```python
from build123d import *

# Parameters (mm, degrees)
BOSS_EXTRUDE1_DEPTH = 10
FILLET1_R           = 2
FILLET2_RADIUS      = 10
FILLET2_LENGTH      = 1.25
FILLET3_R           = 6
SKETCH2_R           = 4.25
CUT_EXTRUDE1_DEPTH  = 29.94740921


with BuildPart() as part:
    # Sketch1 → Boss-Extrude1 (new, symmetric)
    with BuildSketch(Plane.XY):
        Polygon((0, 1.25), (-1.25, 0), (-27.05, 0), (-27.05, -1.25), (0, -1.25), (1.25, 0), (27.05, 0), (27.05, 1.25), align=None)
    extrude(amount=BOSS_EXTRUDE1_DEPTH, both=True)

    # Fillet1
    fillet1_edges = [part.edges().sort_by_distance(p)[0] for p in [
        (-27.05, -0.625, -10),
        (-27.05, -0.625, 10),
    ]]
    fillet(fillet1_edges, radius=FILLET1_R)

    # Fillet2: full round fillet: the end face becomes a half cylinder, R = half its width
    fillet2_face = Plane((27.05, 0.625, 0), x_dir=(0, -1, 0), z_dir=(1, 0, 0))  # on the end face: x along it, z out of the body
    fillet2_slab = fillet2_face.offset(-FILLET2_RADIUS / 2) * Box(FILLET2_LENGTH, 2 * FILLET2_RADIUS, FILLET2_RADIUS, mode=Mode.PRIVATE)  # the body's end, R deep
    fillet2_round = Plane((17.05, 0.625, 0), x_dir=(1, 0, 0), z_dir=(0, -1, 0)) * Cylinder(FILLET2_RADIUS, FILLET2_LENGTH, mode=Mode.PRIVATE)  # its axis R under the face
    add(fillet2_slab - fillet2_round, mode=Mode.SUBTRACT)

    # Fillet3
    # the kernel refuses this fillet: 6 mm, written as the material it takes off along each edge
    with BuildSketch(Plane(origin=(0, -1.25, -16.039298937), x_dir=(-1, 0, 0), z_dir=(0, 0, 1))) as fillet3_piece_1:
        with BuildLine():
            CenterArc((2.415719575, -6), FILLET3_R, 90, 37.658462006)
            Line((-1.25, -1.25), (-1.323314391, -1.155))
            ThreePointArc((-1.323314391, -1.155), (-0.709852814, -0.540147186), (-0.084852814, 0.084852814))
            Line((-0.084852814, 0.084852814), (0, 0.12))
            Line((0, 0.12), (2.415719575, 0.12))
            Line((2.415719575, 0.12), (2.415719575, 0))
        make_face()
    extrude(amount=32.078597873, mode=Mode.SUBTRACT)
    with BuildSketch(Plane(origin=(0, 1.25, 16.039298937), x_dir=(1, 0, 0), z_dir=(0, 0, -1))) as fillet3_piece_2:
        with BuildLine():
            CenterArc((2.415719575, 6), FILLET3_R, 232.341537994, 37.658462006)
            Line((-1.25, 1.25), (-1.323314391, 1.155))
            ThreePointArc((-1.323314391, 1.155), (-0.709852814, 0.540147186), (-0.084852814, -0.084852814))
            Line((-0.084852814, -0.084852814), (0, -0.12))
            Line((0, -0.12), (2.415719575, -0.12))
            Line((2.415719575, -0.12), (2.415719575, 0))
        make_face()
    extrude(amount=32.078597873, mode=Mode.SUBTRACT)

    # Sketch2 → Cut-Extrude1 (cut, through all)
    with BuildSketch(Plane(origin=(0, 1.25, 0), x_dir=(1, 0, 0), z_dir=(0, 1, 0))):
        with Locations(Location((17.05, 0, 0), (0, 0, 270))):
            Circle(SKETCH2_R)
    extrude(amount=-CUT_EXTRUDE1_DEPTH, mode=Mode.SUBTRACT)


solid = part.part
```
Can you work these out from the model? Positions are in its coordinate system, mm. A direction names the side the tool comes from. Give positions to 0.01 mm unless a question says otherwise; leave off trailing zeros. Loops run counter-clockwise (first coordinate to the right, second up) from the corner with the lowest first, then second, coordinate; pieces in that order, holes last. Notation, with made-up numbers: M 56,39 L 66,39 A13 ccw 66,57 Z; hole C 83.25,-2.75 d10. An arc over 180 degrees is marked long. One line per item, written item: value.
(1) Suppose I cut it at B-B on x = 11. List the corners of the cut face in (y, z) for me.
Returned:
outline: M 0,-10 L 1.25,-10 L 1.25,10 L 0,10 Z
(2) We'd pull the mould along Z, two halves only. Please class faces 4 (the face through (-4.3, -0.3, -10)), 5 (the face through (-26.48, -0.63, 9.4)), 6 (the face through (12, 1.25, 0)), 7 (the face through (21.264, 0.634, -0.553)): released by +Z, released by -Z, zero draft, split by the parting line, or undercut.
Returned:
face 4: released by -Z
face 5: released by +Z
face 6: zero draft
face 7: undercut
(3) Will these pins go through, and if not, where does the flat tip stop? pin 1 (1.5 mm diameter, centred on x = -7, z = 5.5, fed in from +Y); pin 2 (12 mm diameter, centred on x = 2, z = 6.5, fed in from -Y).
Returned:
pin 1: y = 0
pin 2: y = -1.25
(4) Suppose I cut it at C-C on z = -5. List the corners of the cut face in (x, y) for me.
Returned:
outline: M -27.05,-1.25 L -2.42,-1.25 A6 ccw 1.25,0 L 25.71,0 L 25.71,1.25 L 2.42,1.25 A6 ccw -1.25,0 L -27.05,0 Z
(5) I need wall thicknesses on line 1 (Y direction, x = -11.5, z = -6.25); line 2 (Y direction, x = 8.5, z = -9); line 3 (X direction, y = 0.65, z = 0). Which ranges of each line are inside material? Lowest first, please.
Returned:
line 1: -1.25 to 0
line 2: 0 to 1.25
line 3: -0.2 to 12.8, 21.3 to 27.05
(6) Suppose I cut it at A-A on z = 0. List the corners of the cut face in (x, y) for me, plus the area to 3 significant figures.
Returned:
outline: M -27.05,-1.25 L -2.42,-1.25 A6 ccw 1.25,0 L 12.8,0 L 12.8,1.25 L 2.42,1.25 A6 ccw -1.25,0 L -27.05,0 Z; M 21.3,0 L 27.05,0 L 27.05,1.25 L 21.3,1.25 Z
area: 57.2 mm^2
(7) Which directions (+Z, -Z, +X, -X, +Y, -Y) give clear straight access to the entire face, cutting with the end or side of a thin tool? Please do faces 1 (the face through (27.048, 0.616, -0.22)), 2 (the face through (-14, 0, 0)), 3 (the face through (11, 0, 0)).
Returned:
face 1: +X, +Y, -Y
face 2: +Z, -Z, -X, +Y
face 3: +Z, -Z, +X, -Y
